Design review of the part built by this model. Coordinates are the model's own, in mm. A direction names the side the tool comes from. Coordinates: 2 decimals unless noted, no trailing zeros. Loops run counter-clockwise (first coordinate to the right, second up) from the corner with the lowest first, then second, coordinate; pieces in that order, holes last. Notation, with made-up numbers: (-3, 35) -> (33, 35) arc R31 ccw to (33, 70) -> close; hole circle Ø11 at (43.5, 37). An arc over 180 degrees is marked (long way). Answer as a JSON object with one key per item and string values.
Solid Edge part; units mm, degrees
sketch "Sketch1" plane through (0, 0, 0) normal (1, 0, 0) x (0, 1, 0)
  line L0 (-30.5556, 21) -> (-30.5556, 65)
  line L1 (-30.5556, 65) -> (-25.5556, 65)
  line L2 (-25.5556, 65) -> (-25.5556, 55)
  line L3 (-25.5556, 55) -> (-5.5556, 55)
  line L4 (-5.5556, 55) -> (-5.5556, 30)
  line L5 (-5.5556, 30) -> (9.4444, 30)
  line L6 (9.4444, 30) -> (9.4444, 21)
  line L7 (9.4444, 21) -> (-30.5556, 21)
  dimension "D1" = 30.5556
  dimension "D2" = 25.5556
  dimension "D3" = 5.5556
  dimension "D4" = 25.5556
  dimension "D5" = 5.5556
revolve "RevolvedProtrusion1" add sketch "Sketch1" angle 360 about axis through (0, -60, 0) along (0, 1, 0)
sketch "Sketch2" plane through (0, -5.5556, 0) normal (0, 1, 0) x (-1, 0, 0)
  line L0 (-4, 40.4732) -> (4, 40.4732)
  line L1 (4, 40.4732) -> (4, -40.4732)
  line L2 (4, -40.4732) -> (-4, -40.4732)
  line L3 (-4, -40.4732) -> (-4, 40.4732)
  dimension "D1" = 4
  dimension "D2" = 4
extrude "Cutout1" cut sketch "Sketch2" along normal blind 383.6956
hole "Hole_2" at (0, 5.0428, 0) direction (1, 0, 0) diameter 5.8 end up to next
hole "Hole_3" at (0, 5.0428, 0) direction (-1, 0, 0) diameter 5.8 end up to next
1) Add section C-C, the plane x = -25. Give the boundary of the cut face in (y, z).
Completed:
{"outline": "(-30.56, -60) -> (-25.56, -60) -> (-25.56, -48.99) -> (-5.56, -48.99) -> (-5.56, -16.58) -> (9.44, -16.58) -> (9.44, 16.58) -> (-5.56, 16.58) -> (-5.56, 48.99) -> (-25.56, 48.99) -> (-25.56, 60) -> (-30.56, 60) -> close; hole circle Ø5.8 at (5.04, 0)"}
2) Add section A-A, the plane x = 0. Give the boundary of the cut face in (y, z), and give its area (3 significant figures).
Completed:
{"outline": "(-30.56, -65) -> (-25.56, -65) -> (-25.56, -55) -> (-5.56, -55) -> (-5.56, -21) -> (-30.56, -21) -> close; (-30.56, 21) -> (-5.56, 21) -> (-5.56, 55) -> (-25.56, 55) -> (-25.56, 65) -> (-30.56, 65) -> close", "area": "1,800 mm²"}
3) For faces 4 (the flat face through (-4, 2, -25)), 5 (the cylindrical face through (29.994, 2.049, 0.604)), 6 (the flat face through (14.7, -25.556, -53.3)), list the 3-axis set-ups (+Z, -Z, +X, -X, +Y, -Y) from which the entire face can be reached by the end or side of a thin tool; tool diameter is ignored.
Completed:
{"face 4": "+Z, -Z, +Y", "face 5": "+X, +Y", "face 6": "+Y"}
4) Add section B-B, the plane z = 0. Give the boundary of the cut face in (x, y), and give its area (3 significant figures).
Completed:
{"outline": "(-65, -30.56) -> (-21, -30.56) -> (-21, 2.14) -> (-30, 2.14) -> (-30, -5.56) -> (-55, -5.56) -> (-55, -25.56) -> (-65, -25.56) -> close; (-30, 7.94) -> (-21, 7.94) -> (-21, 9.44) -> (-30, 9.44) -> close; (21, -30.56) -> (65, -30.56) -> (65, -25.56) -> (55, -25.56) -> (55, -5.56) -> (30, -5.56) -> (30, 2.14) -> (21, 2.14) -> close; (21, 7.94) -> (30, 7.94) -> (30, 9.44) -> (21, 9.44) -> close", "area": "1,970 mm²"}
5) Clearance check with flat-ended pins moving along their axes: pin 1 Ø4 at (x, y) = (-11, -3) entering from -Z; pin 2 Ø4 at (y, z) = (-3.5, -15) entering from -X; pin 3 Ø10 at (y, z) = (-1.5, 25.5) entering from +X. State where each tip first meets the part, or that it passes through.
Completed:
{"pin 1": "z = -28.62", "pin 2": "x = -27.04", "pin 3": "x = 50.15"}
6) The part is to be moulded in two halves that separate along Z. For faces 1 (the cylindrical face through (-29.994, 2.049, -0.604)), 2 (the cylindrical face through (-25.335, 7.918, 0.378)), 3 (the flat face through (4, 2, -25)), say which applies: pulls with the +Z half, pulls with the -Z half, needs draft (parallel to the pull), parting line crosses it, or undercut.
Completed:
{"face 1": "parting line crosses it", "face 2": "undercut", "face 3": "needs draft"}
7) Wall thickness on probe 1 along Y at (x, z) = (24, 0); probe 2 along X at (y, z) = (-16, 0); probe 3 along Y at (x, z) = (-31.5, -24): over which ranges is each line inside the solid? List them lowest first.
Completed:
{"probe 1": "-30.56 to 2.14, 7.94 to 9.44", "probe 2": "-55 to -21, 21 to 55", "probe 3": "-30.56 to -5.56"}
8) Add section D-D, the plane z = -49.5. Give the boundary of the cut face in (x, y).
Completed:
{"outline": "(-42.13, -30.56) -> (42.13, -30.56) -> (42.13, -25.56) -> (23.97, -25.56) -> (23.97, -5.56) -> (-23.97, -5.56) -> (-23.97, -25.56) -> (-42.13, -25.56) -> close"}
